from build123d import *

# Parameters (mm, degrees)
F1_DEPTH = 12.7


with BuildPart() as f1:
    # F0 (on Top) → F1 (new body)
    with BuildSketch(Plane.XY):
        with BuildLine():
            Line((166.6875, -333.375), (166.6875, -166.6875))
            Line((166.6875, -166.6875), (50.8, -166.6875))
            ThreePointArc((50.8, -166.6875), (0, -217.4875), (-50.8, -166.6875))
            Line((-50.8, -166.6875), (-166.6875, -166.6875))
            Line((-166.6875, -166.6875), (-166.6875, -333.375))
            Line((-166.6875, -333.375), (-19.05, -333.375))
            Line((-19.05, -333.375), (-19.05, -317.5))
            Line((-19.05, -317.5), (19.05, -317.5))
            Line((19.05, -317.5), (19.05, -333.375))
            Line((19.05, -333.375), (166.6875, -333.375))
        make_face()
        with BuildLine():
            Line((50.8, 166.6875), (166.6875, 166.6875))
            Line((166.6875, 166.6875), (166.6875, 333.375))
            Line((166.6875, 333.375), (19.05, 333.375))
            Line((19.05, 333.375), (19.05, 317.5))
            Line((19.05, 317.5), (-19.05, 317.5))
            Line((-19.05, 317.5), (-19.05, 333.375))
            Line((-19.05, 333.375), (-166.6875, 333.375))
            Line((-166.6875, 333.375), (-166.6875, 166.6875))
            Line((-166.6875, 166.6875), (-50.8, 166.6875))
            ThreePointArc((-50.8, 166.6875), (0, 217.4875), (50.8, 166.6875))
        make_face()
        with BuildLine():
            Line((50.8, -166.6875), (166.6875, -166.6875))
            Line((166.6875, -166.6875), (166.6875, -19.05))
            Line((166.6875, -19.05), (150.8125, -19.05))
            Line((150.8125, -19.05), (150.8125, 19.05))
            Line((150.8125, 19.05), (166.6875, 19.05))
            Line((166.6875, 19.05), (166.6875, 166.6875))
            Line((166.6875, 166.6875), (50.8, 166.6875))
            ThreePointArc((50.8, 166.6875), (0, 115.8875), (-50.8, 166.6875))
            Line((-50.8, 166.6875), (-166.6875, 166.6875))
            Line((-166.6875, 166.6875), (-166.6875, 19.05))
            Line((-166.6875, 19.05), (-150.8125, 19.05))
            Line((-150.8125, 19.05), (-150.8125, -19.05))
            Line((-150.8125, -19.05), (-166.6875, -19.05))
            Line((-166.6875, -19.05), (-166.6875, -166.6875))
            Line((-166.6875, -166.6875), (-50.8, -166.6875))
            ThreePointArc((-50.8, -166.6875), (0, -115.8875), (50.8, -166.6875))
        make_face()
    extrude(amount=F1_DEPTH)


solid = f1.part
The model under review builds one solid part; all positions refer to its coordinate system, in mm. A direction names the side the tool comes from. Give positions to 0.01 mm unless a question says otherwise; leave off trailing zeros. Write each loop counter-clockwise with the first axis right and the second up, starting at its lowest first coordinate (ties: lowest second). Pieces come first, ordered by that corner, then holes.
1. Wall thickness on L1, parallel to Y at x = 0, z = 3; L2, parallel to Y at x = -18, z = 9.25; L3, parallel to X at y = 119.5, z = 8.5: over which ranges is each line inside the solid? List them lowest first.
2. Tool access review of faces 4 (the flat face through (166.688, -178, 6)), 5 (the flat face through (-159, 19.05, 6)), 6 (the flat face through (150.812, 0, 6)), 7 (the flat face through (-19.05, 325, 6)), 8 (the flat face through (-19.05, -326, 6)): name each direction out of +Z, -Z, +X, -X, +Y, -Y from which nothing blocks a thin tool from reaching the whole face with its end or side.
3. Add section D-D, the plane x = -36. Write out the cut boundary in (y, z) (3 decimals).
4. Add section C-C, the plane y = -200.5. Write out the cut boundary in (x, z), plus the area to 3 significant figures.
5. Draft analysis for pull direction X (two halves, no side actions). For faces 1 (the flat face through (0, 317.5, 6)), 2 (the flat face through (-166.688, -174, 6)), 3 (the flat face through (159, 19.05, 6)), state which applies: +X half, -X half, draft (parallel to the pull), parting line (faces both ways), or undercut.
6. Add section B-B, the plane z = 4.5. Count the separate pieces of the cut face and the enclosed holes in it, plus the area to 3 significant figures.
7. Add section A-A, the plane x = 0. Write out the cut boundary in (y, z), plus the area to 3 significant figures.
Worked answers:
1. L1: y = -317.5 to -217.49, -115.89 to 115.89, 217.49 to 317.5
1. L2: y = -317.5 to -214.19, -119.18 to 119.18, 214.19 to 317.5
1. L3: x = -166.69 to -18.81, 18.81 to 166.69
2. face 4: +Z, -Z, +X, +Y, -Y
2. face 5: +Z, -Z, -X
2. face 6: +Z, -Z, +X
2. face 7: +Z, -Z, +Y
2. face 8: +Z, -Z, -Y
3. outline: (-333.375, 0) - (-202.529, 0) - (-202.529, 12.7) - (-333.375, 12.7) - close; (-130.846, 0) - (130.846, 0) - (130.846, 12.7) - (-130.846, 12.7) - close; (202.529, 0) - (333.375, 0) - (333.375, 12.7) - (202.529, 12.7) - close
4. outline: (-166.69, 0) - (-37.91, 0) - (-37.91, 12.7) - (-166.69, 12.7) - close; (37.91, 0) - (166.69, 0) - (166.69, 12.7) - (37.91, 12.7) - close
4. area: 3,270 mm2
5. face 1: undercut
5. face 2: -X half
5. face 3: draft
6. separate pieces: 1
6. enclosed holes: 2
6. area: 204,000 mm2
7. outline: (-317.5, 0) - (-217.49, 0) - (-217.49, 12.7) - (-317.5, 12.7) - close; (-115.89, 0) - (115.89, 0) - (115.89, 12.7) - (-115.89, 12.7) - close; (217.49, 0) - (317.5, 0) - (317.5, 12.7) - (217.49, 12.7) - close
7. area: 5,480 mm2
